Can you work these out from the model? Positions are in its coordinate system, mm. Round coordinates to 2 decimals unless told otherwise and drop trailing zeros. Order: outer loops, then holes, each group sorted by start corner. A loop starts at its lowest first (then second) coordinate and runs counter-clockwise, first axis right, second up. Notation, with made-up numbers: (65.25, 32) - (80.25, 32) arc R21 cw to (80.25, 63) - close; hole circle Ø11 at (52, 57). An arc over 180 degrees is marked (long way). Write item = value, one per line.
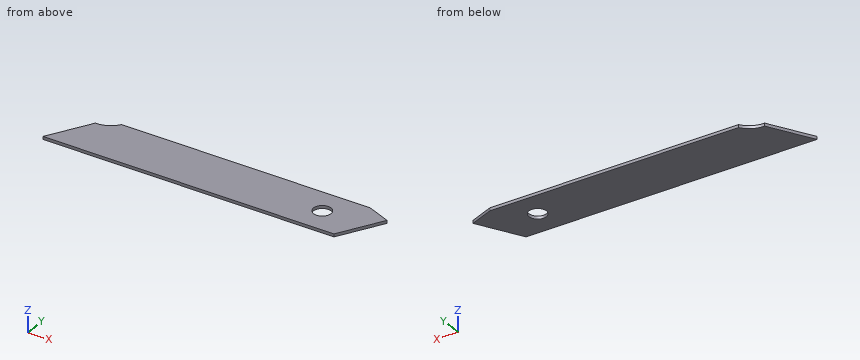
from build123d import *

# Parameters (mm, degrees)
SKETCH1_R           = 3
BOSS_EXTRUDE1_DEPTH = 1


with BuildPart() as part:
    # Sketch1 → Boss-Extrude1 (new body)
    with BuildSketch(Plane.XY):
        with BuildLine():
            Line((8.399507831, 14.548374322), (0, 0))
            Line((0, 0), (100, 0))
            Line((100, 0), (108.516319797, 14.750698581))
            Line((108.516319797, 14.750698581), (100.60138269, 18))
            Line((100.60138269, 18), (15.167032503, 18))
            ThreePointArc((15.167032503, 18), (12.241054752, 15.376619242), (8.399507831, 14.548374322))
        make_face()
        with Locations((90.015809824, 9.06195858)):
            Circle(SKETCH1_R, mode=Mode.SUBTRACT)
    extrude(amount=BOSS_EXTRUDE1_DEPTH)


solid = part.part
(1) If we section it at B-B (z = 0.5): Write out the boundary of the cut face in (x, y).
Computed:
outline = (0, 0) - (100, 0) - (108.52, 14.75) - (100.6, 18) - (15.17, 18) arc R7.66 cw to (8.4, 14.55) - close; hole circle Ø6 at (90.02, 9.06)
(2) If we section it at C-C (y = 16.25): Write out the boundary of the cut face in (x, z), plus the area to 3 significant figures.
Computed:
outline = (13.58, 0) - (104.86, 0) - (104.86, 1) - (13.58, 1) - close
area = 91.3 mm^2
(3) If I drill on line 1 (X direction, y = 10.25, z = 0.25); line 2 (X direction, y = 9.75, z = 0.35); line 3 (X direction, y = 2.5, z = 0.3), over which ranges is the centre line in solid material (lowest first)? Write a range as from..to.
Computed:
line_1 = 5.92..87.26, 92.77..105.92
line_2 = 5.63..87.1, 92.94..105.63
line_3 = 1.44..101.44
(4) If we section it at A-A (y = 8): Write out the boundary of the cut face in (x, z), plus the area to 3 significant figures.
Computed:
outline = (4.62, 0) - (87.21, 0) - (87.21, 1) - (4.62, 1) - close; (92.82, 0) - (104.62, 0) - (104.62, 1) - (92.82, 1) - close
area = 94.4 mm^2
(5) Will this pin go through, and if not, where does the flat tip stop? P1, Ø9.5, axis at x = 90.02, y = 9.06, coming from the +Z side.
Computed:
P1 = 1
